```python
from build123d import *

# Parameters (mm, degrees)
SKETCH_1_W          = 30
SKETCH_1_H          = 17.5
SKETCH_1_W_2        = 8.956326716
SKETCH_1_H_2        = 12.5
EXTRUDE_1_DEPTH     = 17.6
FILLET_1_R          = 1
SKETCH_3_W          = 10.521836642
SKETCH_3_H          = 17.5
EXTRUDE_2_DEPTH     = 2.1
FILLET_2_R          = 2
SKETCH_4_R          = 2.1
CUT_EXTRUDE_1_DEPTH = 10


with BuildPart() as part:
    # 草图1 → 凸台-拉伸1 (new body)
    with BuildSketch(Plane.XY):
        Rectangle(SKETCH_1_W, SKETCH_1_H)
        Polygon((11.760918321, 3.05), (8.239081679, 3.05), (6.478163358, 0), (8.239081679, -3.05), (11.760918321, -3.05), (13.521836642, 0), align=None, mode=Mode.SUBTRACT)
        Polygon((-11.760918321, 3.05), (-13.521836642, 0), (-11.760918321, -3.05), (-8.239081679, -3.05), (-6.478163358, 0), (-8.239081679, 3.05), align=None, mode=Mode.SUBTRACT)
        Rectangle(SKETCH_1_W_2, SKETCH_1_H_2, mode=Mode.SUBTRACT)
    extrude(amount=EXTRUDE_1_DEPTH)

    # 圆角1
    fillet_1_edges = [part.edges().sort_by_distance(p)[0] for p in [
        (4.478163358, -6.25, 8.8),
        (4.478163358, 6.25, 8.8),
        (-4.478163358, 6.25, 8.8),
        (-4.478163358, -6.25, 8.8),
    ]]
    fillet(fillet_1_edges, radius=FILLET_1_R)

    # 草图3 → 凸台-拉伸2 (add)
    with BuildSketch(Plane(origin=(0, 0, 0), x_dir=(-1, 0, 0), z_dir=(0, 0, -1))):
        with Locations((-9.739081679, 0)):
            Rectangle(SKETCH_3_W, SKETCH_3_H)
        with Locations((9.739081679, 0)):
            Rectangle(SKETCH_3_W, SKETCH_3_H)
    extrude(amount=-EXTRUDE_2_DEPTH)

    # 圆角2
    fillet_2_edges = [part.edges().sort_by_distance(p)[0] for p in [
        (15, -8.75, 8.8),
        (-15, -8.75, 8.8),
        (-15, 8.75, 8.8),
        (15, 8.75, 8.8),
    ]]
    fillet(fillet_2_edges, radius=FILLET_2_R)

    # 草图4 → 切除-拉伸1 (cut)
    with BuildSketch(Plane.XY.offset(2.1)):
        with Locations((10, 0)):
            Circle(SKETCH_4_R)
        with Locations((-10, 0)):
            Circle(SKETCH_4_R)
    extrude(amount=-CUT_EXTRUDE_1_DEPTH, mode=Mode.SUBTRACT)


solid = part.part
```
Geometry: final body of the model. Coordinates: model frame, mm. A direction names the side the tool comes from. Round coordinates to 2 decimals unless told otherwise and drop trailing zeros. Loops run counter-clockwise (first coordinate to the right, second up) from the corner with the lowest first, then second, coordinate; pieces in that order, holes last.
Item 1: Section D-D, the plane x = 9.5. Output: boundary loops of the cut face in (y, z).
Checked values:
outline: (-8.75, 0) - (-2.04, 0) - (-2.04, 2.1) - (-3.05, 2.1) - (-3.05, 17.6) - (-8.75, 17.6) - close; (2.04, 0) - (8.75, 0) - (8.75, 17.6) - (3.05, 17.6) - (3.05, 2.1) - (2.04, 2.1) - close
Item 2: Section C-C, the plane y = -4.5. Output: boundary loops of the cut face in (x, z).
Checked values:
outline: (-15, 0) - (-4.48, 0) - (-4.48, 17.6) - (-15, 17.6) - close; (4.48, 0) - (15, 0) - (15, 17.6) - (4.48, 17.6) - close
Item 3: Reachability of faces 1 (the cylindrical face through (-4.18, -5.96, 8.92)), 2 (the cylindrical face through (14.43, -8.15, 8.68)), 3 (the flat face through (-7.371, -1.546, 9.742)) from +Z, -Z, +X, -X, +Y, -Y: full face, straight path, thin tool, end or side. Return the list, or none.
Checked values:
face 1: +Z, -Z
face 2: +Z, -Z, +X, -Y
face 3: +Z
Item 4: Section A-A, the plane x = -10. Output: boundary loops of the cut face in (y, z), plus the area to 3 significant figures.
Checked values:
outline: (-8.75, 0) - (-2.1, 0) - (-2.1, 2.1) - (-3.05, 2.1) - (-3.05, 17.6) - (-8.75, 17.6) - close; (2.1, 0) - (8.75, 0) - (8.75, 17.6) - (3.05, 17.6) - (3.05, 2.1) - (2.1, 2.1) - close
area: 205 mm2
Item 5: Contact query for a flat-ended pin moving along its axis: P1, Ø3, axis at x = 11, y = -2, coming from the -Z side. Output: stop coordinate, or through.
Checked values:
P1: stops at z = 0
Item 6: Mould query, pull axis X, two halves, no side actions, for faces 4 (the cylindrical face through (14.43, 8.15, 8.68)), 5 (the cylindrical face through (-14.43, 8.15, 8.92)), 6 (the flat face through (0, 6.25, 9)). Classes: released by +X, released by -X, zero draft, split by the parting line, or undercut.
Checked values:
face 4: released by +X
face 5: released by -X
face 6: undercut
Item 7: Section B-B, the plane z = 12.75. Output: boundary loops of the cut face in (x, y).
Checked values:
outline: (-15, -6.75) arc R2 ccw to (-13, -8.75) - (13, -8.75) arc R2 ccw to (15, -6.75) - (15, 6.75) arc R2 ccw to (13, 8.75) - (-13, 8.75) arc R2 ccw to (-15, 6.75) - close; hole (-13.52, 0) - (-11.76, -3.05) - (-8.24, -3.05) - (-6.48, 0) - (-8.24, 3.05) - (-11.76, 3.05) - close; hole (-4.48, -5.25) arc R1 ccw to (-3.48, -6.25) - (3.48, -6.25) arc R1 ccw to (4.48, -5.25) - (4.48, 5.25) arc R1 ccw to (3.48, 6.25) - (-3.48, 6.25) arc R1 ccw to (-4.48, 5.25) - close; hole (6.48, 0) - (8.24, -3.05) - (11.76, -3.05) - (13.52, 0) - (11.76, 3.05) - (8.24, 3.05) - close
Item 8: Line query: L1, parallel to Y at x = -11.5, z = 2.25; L2, parallel to Y at x = -0.25, z = 6; L3, parallel to X at y = 3.25, z = 2.5. Output: solid intervals per line, ascending.
Checked values:
L1: y = -8.75 to -3.05, 3.05 to 8.75
L2: y = -8.75 to -6.25, 6.25 to 8.75
L3: x = -15 to -4.48, 4.48 to 15
